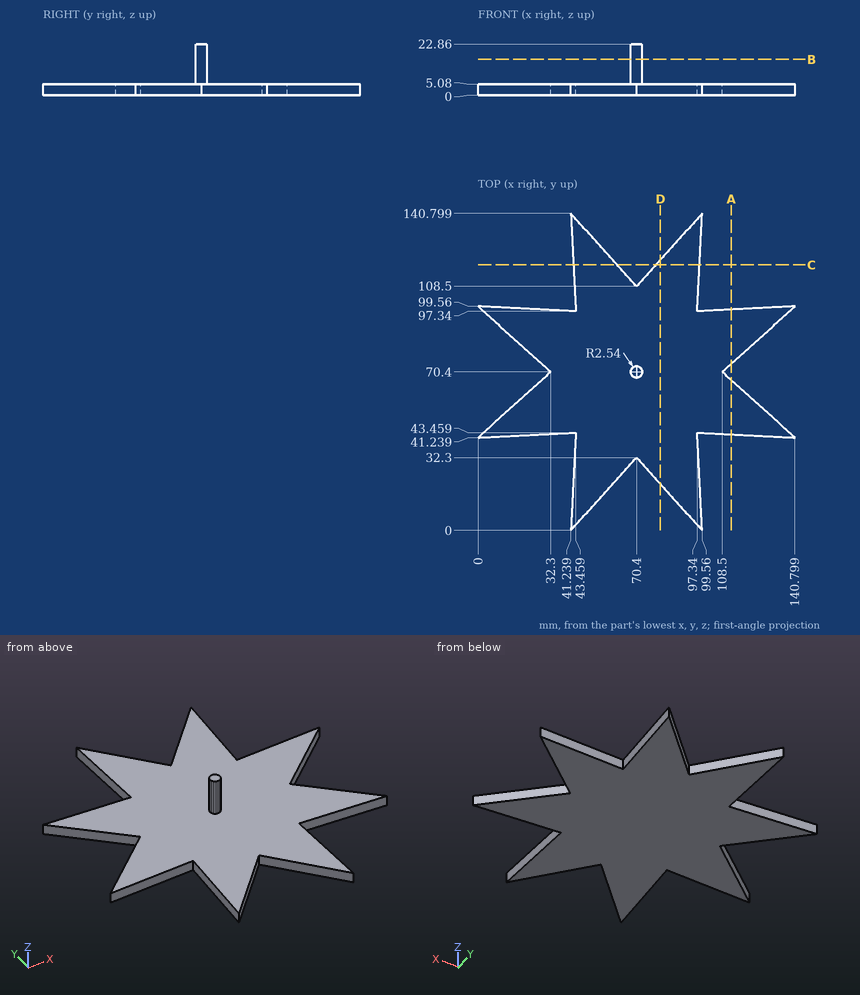
Input: dimensioned drawing with shaded views. Units: mm. Origin: part minimum x, y, z. Coordinates: 2 decimals unless noted, no trailing zeros. Loops run counter-clockwise (first coordinate to the right, second up) from the corner with the lowest first, then second, coordinate; pieces in that order, holes last. Notation, with made-up numbers: M -30.5,77 L -6.5,77 A11 ccw -6.5,84 Z; hole C 64.5,43 d7. An arc over 180 degrees is marked long. One line per item, written item: value. Start each with the question number.
1) Cut plane A-A (x = 112.5). Return loops of the section in (y, z) (1 decimal).
2) Material intervals for L1, parallel to Z at x = 65.5, y = 111.5; L2, parallel to X at y = 112.5, z = 1.5 (1 decimal); L3, parallel to X at y = 10, z = 2, sorted ascending. Write a range as from..to.
3) Pin query (flat end, axial travel): P1, Ø12, axis at x = 35, z = 2.5, coming from the -Y side; P2, Ø6, axis at x = 106.5, y = 63.5, coming from the +Z side; P3, Ø12, axis at x = 24.5, z = 4.5, coming from the +Y side (1 decimal). Return the tip coordinate at first contact, or that it passes through.
4) Cut plane B-B (z = 16). Return loops of the section in (x, y) (1 decimal), then the cut area to 3 significant figures.
5) Cut plane C-C (y = 118). Return loops of the section in (x, z) (1 decimal).
6) Cut plane D-D (x = 81). Return loops of the section in (y, z).
Evaluation:
1. outline: M 42.7,0 L 66.8,0 L 66.8,5.1 L 42.7,5.1 Z; M 74,0 L 98.1,0 L 98.1,5.1 L 74,5.1 Z
2. L1: 0..5.08
2. L2: 42.7..66.8, 74..98.1
2. L3: 41.75..50.27, 90.53..99.05
3. P1: y = 42.72
3. P2: z = 5.08
3. P3: y = 98.6
4. outline: C 70.4,70.4 d5.1
4. area: 20.3 mm^2
5. outline: M 42.4,0 L 61.8,0 L 61.8,5.1 L 42.4,5.1 Z; M 79,0 L 98.4,0 L 98.4,5.1 L 79,5.1 Z
6. outline: M 20.56,0 L 120.24,0 L 120.24,5.08 L 20.56,5.08 Z
